Build history of the part. All positions in model axes, mm. A direction names the side the tool comes from. Round coordinates to 2 decimals unless told otherwise and drop trailing zeros. Write each loop counter-clockwise with the first axis right and the second up, starting at its lowest first coordinate (ties: lowest second). Pieces come first, ordered by that corner, then holes. Notation, with made-up numbers: (20.25, 55.25) -> (75.25, 55.25) arc R19 ccw to (75.25, 78.25) -> close; hole circle Ø2 at (50.5, -4.5). An arc over 180 degrees is marked (long way). Answer in a Markdown table with one row per item. Add a question column.
from build123d import *

# Parameters (mm, degrees)
SKETCH_R    = 1.6
PAD_DEPTH   = 1
FILLET_R    = 0.5
FILLET001_R = 0.5
FILLET002_R = 0.5
FILLET003_R = 0.5
FILLET004_R = 0.5
FILLET005_R = 0.5


with BuildPart() as part:
    # Sketch → Pad (new body)
    with BuildSketch(Plane.XY):
        with BuildLine():
            Line((-13.5, 9.5), (-3.864318, 9.5))
            ThreePointArc((0.864318, 9.5), (-1.5, 13.8), (-3.864318, 9.5))
            Line((0.864318, 9.5), (13.5, 9.5))
            Line((13.5, 9.5), (13.5, 2.297825))
            ThreePointArc((13.5, -2.297825), (17.9, 0), (13.5, 2.297825))
            Line((13.5, -2.297825), (13.5, -9.5))
            Line((13.5, -9.5), (1.098076, -9.5))
            ThreePointArc((1.098076, -9.5), (-1.5, -5), (-4.098076, -9.5))
            Line((-4.098076, -9.5), (-13.5, -9.5))
            Line((-13.5, -9.5), (-13.5, -2.537716))
            ThreePointArc((-13.5, -2.537716), (-8.9, 0), (-13.5, 2.537716))
            Line((-13.5, 2.537716), (-13.5, 9.5))
        make_face()
        with Locations((-1.5, 11)):
            Circle(SKETCH_R, mode=Mode.SUBTRACT)
        with Locations((15.1, 0)):
            Circle(SKETCH_R, mode=Mode.SUBTRACT)
    extrude(amount=PAD_DEPTH)

    # Fillet
    fillet_edges = [part.edges().sort_by_distance(p)[0] for p in [
        (-3.864318, 9.5, 0.5),
    ]]
    fillet(fillet_edges, radius=FILLET_R)

    # Fillet001
    fillet001_edges = [part.edges().sort_by_distance(p)[0] for p in [
        (0.864318, 9.5, 0.5),
    ]]
    fillet(fillet001_edges, radius=FILLET001_R)

    # Fillet002
    fillet002_edges = [part.edges().sort_by_distance(p)[0] for p in [
        (13.5, 2.297825, 0.5),
    ]]
    fillet(fillet002_edges, radius=FILLET002_R)

    # Fillet003
    fillet003_edges = [part.edges().sort_by_distance(p)[0] for p in [
        (13.5, -2.297825, 0.5),
    ]]
    fillet(fillet003_edges, radius=FILLET003_R)

    # Fillet004
    fillet004_edges = [part.edges().sort_by_distance(p)[0] for p in [
        (-4.098076, -9.5, 0.5),
    ]]
    fillet(fillet004_edges, radius=FILLET004_R)

    # Fillet005
    fillet005_edges = [part.edges().sort_by_distance(p)[0] for p in [
        (1.098076, -9.5, 0.5),
        (-13.5, -2.537716, 0.5),
        (-13.5, 2.537716, 0.5),
    ]]
    fillet(fillet005_edges, radius=FILLET005_R)


solid = part.part
(1) Drop flat-ended pins along their axis: P1, Ø0.5, axis at x = -8.5, z = 0.5, coming from the +Y side; P2, Ø5, axis at x = -1.5, y = -8, coming from the -Z side. Give the stop position or say it passes through.
(2) Saw through at C-C (z = 0.55). List the corners of the cut face in (x, y).
(3) Which spindle directions (+Z, -Z, +X, -X, +Y, -Y) get a long thin tool onto all of the face, cutting with end or side? Do faces 1 (the face through (13.5, 6.4, 0.5)), 2 (the face through (-9.1, 9.5, 0.5)), 3 (the face through (13.5, -6.3, 0.5)). Say none if no direction does.
(4) Saw through at B-B (y = -8). List the corners of the cut face in (x, z).
(5) Probe line 1 along Y through (x, z) = (-12, 0.25); line 2 along Y through (x, z) = (-1.5, 0.4); line 3 along Y through (x, z) = (9.5, 0.85). List the from-to ranges inside material, lowest first.
(6) Saw through at D-D (y = -4.25). List the corners of the cut face in (x, z).
(7) Saw through at A-A (x = -11.9). List the corners of the cut face in (y, z).
Answer sheet:
| question | item | result |
|---|---|---|
| 1 | P1 | stops at y = 9.5 |
| 1 | P2 | passes through |
| 2 | outline | (-13.5, -9.5) -> (-4.85, -9.5) arc R0.5 ccw to (-4.37, -8.86) arc R3 cw (long way) to (1.37, -8.86) arc R0.5 ccw to (1.85, -9.5) -> (13.5, -9.5) -> (13.5, -3.11) arc R0.5 cw to (14.17, -2.64) arc R2.8 ccw (long way) to (14.17, 2.64) arc R0.5 cw to (13.5, 3.11) -> (13.5, 9.5) -> (1.64, 9.5) arc R0.5 cw to (1.17, 10.15) arc R2.8 ccw (long way) to (-4.17, 10.15) arc R0.5 cw to (-4.64, 9.5) -> (-13.5, 9.5) -> (-13.5, 3.32) arc R0.5 ccw to (-12.84, 2.85) arc R3 cw (long way) to (-12.84, -2.85) arc R0.5 ccw to (-13.5, -3.32) -> close; hole circle Ø3.2 at (-1.5, 11); hole circle Ø3.2 at (15.1, 0) |
| 3 | face 1 | +Z, -Z, +X, +Y |
| 3 | face 2 | +Z, -Z, -X, +Y |
| 3 | face 3 | +Z, -Z, +X, -Y |
| 4 | outline | (-13.5, 0) -> (-4.5, 0) -> (-4.5, 1) -> (-13.5, 1) -> close; (1.5, 0) -> (13.5, 0) -> (13.5, 1) -> (1.5, 1) -> close |
| 5 | line 1 | y = -9.5 to -3, 3 to 9.5 |
| 5 | line 2 | y = -5 to 9.4, 12.6 to 13.8 |
| 5 | line 3 | y = -9.5 to 9.5 |
| 6 | outline | (-13.5, 0) -> (13.5, 0) -> (13.5, 1) -> (-13.5, 1) -> close |
| 7 | outline | (-9.5, 0) -> (-3, 0) -> (-3, 1) -> (-9.5, 1) -> close; (3, 0) -> (9.5, 0) -> (9.5, 1) -> (3, 1) -> close |
